from build123d import *

# Parameters (mm, degrees)
SKETCH_1_W          = 240
SKETCH_1_H          = 55
EXTRUDE_1_DEPTH     = 1
CHAMFER_1_SIZE      = 10
SKETCH_2_R          = 2.1
SKETCH_2_R_2        = 1.6
CUT_EXTRUDE_1_DEPTH = 10


with BuildPart() as part:
    # 草图1 → 凸台-拉伸1 (new body)
    with BuildSketch(Plane(origin=(0, 0, 0), x_dir=(1, 0, 0), z_dir=(0, 1, 0))):
        with Locations((120, 27.5)):
            Rectangle(SKETCH_1_W, SKETCH_1_H)
    extrude(amount=EXTRUDE_1_DEPTH)

    # 倒角1
    chamfer_1_edges = [part.edges().sort_by_distance(p)[0] for p in [
        (0, 0.5, -55),
        (240, 0.5, -55),
        (240, 0.5, 0),
        (0, 0.5, 0),
    ]]
    chamfer(chamfer_1_edges, length=CHAMFER_1_SIZE)

    # 草图2 → 切除-拉伸1 (cut)
    with BuildSketch(Plane.XZ):
        with Locations(Location((195, -43, 0), (0, 0, 270))):
            Circle(SKETCH_2_R)
        with Locations(Location((45, -43, 0), (0, 0, 270))):
            Circle(SKETCH_2_R)
        with Locations(Location((235, -27.5, 0), (0, 0, 270))):
            Circle(SKETCH_2_R_2)
        with Locations(Location((5, -27.5, 0), (0, 0, 270))):
            Circle(SKETCH_2_R_2)
        with Locations(Location((20, -5, 0), (0, 0, 270))):
            Circle(SKETCH_2_R_2)
        with Locations(Location((60, -5, 0), (0, 0, 270))):
            Circle(SKETCH_2_R_2)
        with Locations(Location((100, -5, 0), (0, 0, 270))):
            Circle(SKETCH_2_R_2)
        with Locations(Location((140, -5, 0), (0, 0, 270))):
            Circle(SKETCH_2_R_2)
        with Locations(Location((180, -5, 0), (0, 0, 270))):
            Circle(SKETCH_2_R_2)
        with Locations(Location((220, -5, 0), (0, 0, 270))):
            Circle(SKETCH_2_R_2)
        with Locations(Location((40, -5, 0), (0, 0, 270))):
            Circle(SKETCH_2_R_2)
        with Locations(Location((120, -5, 0), (0, 0, 270))):
            Circle(SKETCH_2_R_2)
        with Locations(Location((200, -5, 0), (0, 0, 270))):
            Circle(SKETCH_2_R_2)
    extrude(amount=-CUT_EXTRUDE_1_DEPTH, mode=Mode.SUBTRACT)


solid = part.part
Model file for the job. Use its own axes, mm. Round coordinates to 2 decimals unless told otherwise and drop trailing zeros. Order: outer loops, then holes, each group sorted by start corner. A loop starts at its lowest first (then second) coordinate and runs counter-clockwise, first axis right, second up.
(1) Pull direction Z, two halves, no side cores. Call faces 1 (the face through (235.1, 0.5, -5.1)), 2 (the face through (42.95, 0.49, -42.54)), 3 (the face through (5.1, 0.5, -50.1)): released by +Z, released by -Z, zero draft, split by the parting line, or undercut.
(2) Drill centre lines: line 1 (Z direction, x = 180, y = 0.2); line 2 (Z direction, x = 220.5, y = 0.15); line 3 (X direction, y = 0.85, z = -50). Where is each one in solid material? Low to high.
(3) Band-saw the part on A-A (x = 45). List the corners of the cut face in (y, z), then the cut area to 3 significant figures.
(4) Band-saw the part on C-C (z = -43). List the corners of the cut face in (x, y), then the cut area to 3 significant figures.
(5) Band-saw the part on B-B (y = 0.2). Give the number of separate pieces and of enclosed holes in the cut face, then the cut area to 3 significant figures.
Verdict:
1. face 1: released by +Z
1. face 2: undercut
1. face 3: released by -Z
2. line 1: z = -55 to -6.6, -3.4 to 0
2. line 2: z = -55 to -6.52, -3.48 to 0
2. line 3: x = 5 to 235
3. outline: (0, -55) - (1, -55) - (1, -45.1) - (0, -45.1) - close; (0, -40.9) - (1, -40.9) - (1, 0) - (0, 0) - close
3. area: 50.8 mm2
4. outline: (0, 0) - (42.9, 0) - (42.9, 1) - (0, 1) - close; (47.1, 0) - (192.9, 0) - (192.9, 1) - (47.1, 1) - close; (197.1, 0) - (240, 0) - (240, 1) - (197.1, 1) - close
4. area: 232 mm2
5. separate pieces: 1
5. enclosed holes: 13
5. area: 12,900 mm2
